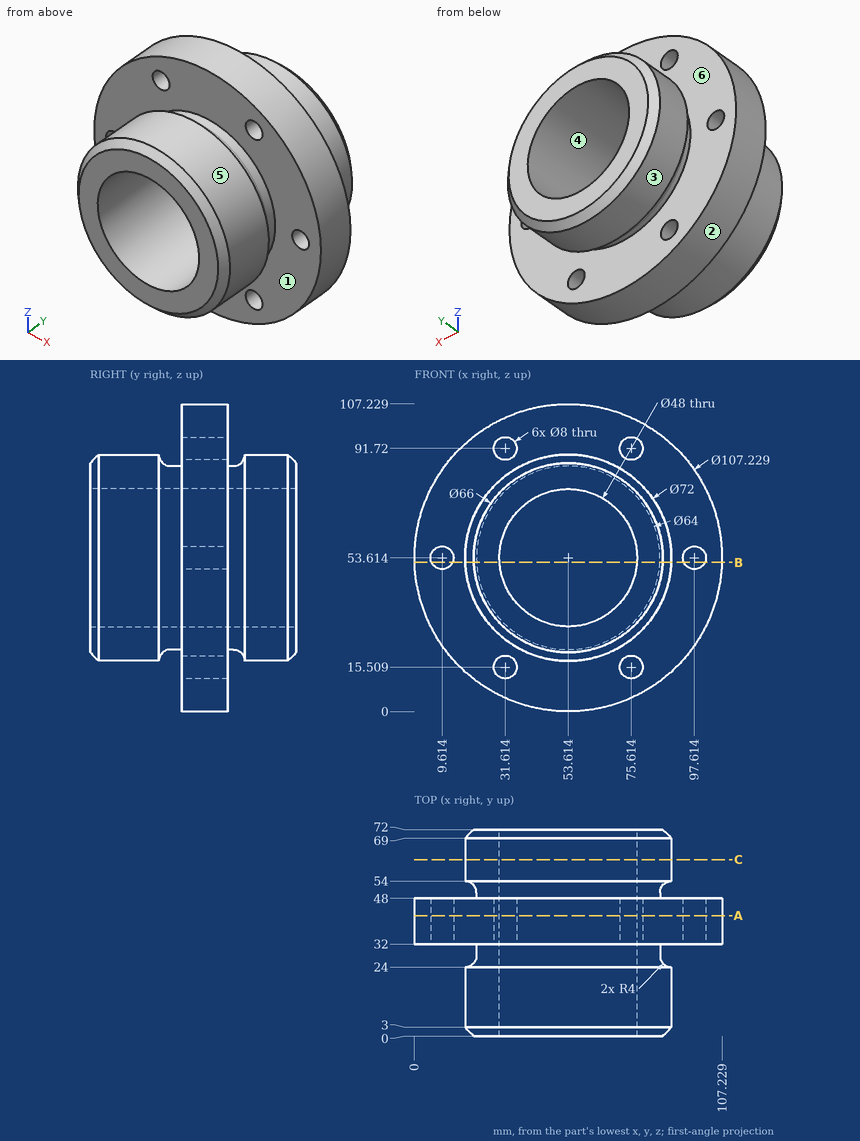
Answer from the drawing. Dimensions are ordinates in mm from the lowest x, y and z of the part. A direction names the side the tool comes from. Coordinates: 2 decimals unless noted, no trailing zeros. Loops run counter-clockwise (first coordinate to the right, second up) from the corner with the lowest first, then second, coordinate; pieces in that order, holes last. Notation, with made-up numbers: (69, 56.25) -> (85, 56.25) arc R21 cw to (85, 70.25) -> close; hole circle Ø3 at (83, 54). An arc over 180 degrees is marked (long way). Return JSON: item names as keys, results as strings.
Item 1: Find the intervals of material crossed by probe 1 along Z at (x, y) = (33, 33) (1 decimal); probe 2 along Y at (x, z) = (9.5, 60.5); probe 3 along X at (y, z) = (7.5, 46.5) (1 decimal), in increasing order.
Answers:
{"probe 1": "z = 4.1 to 11.8, 19.3 to 41.3, 65.9 to 88, 95.5 to 103.1", "probe 2": "y = 32 to 48", "probe 3": "x = 18.3 to 30.7, 76.5 to 88.9"}
Item 2: For the marked faces 1, 2 and 3, determine the directions among +Z, -Z, +X, -X, +Y, -Y from which every point of the face is accessible in a straight line to the end or side of a thin tool.
Answers:
{"face 1": "none", "face 2": "+Y, -Y", "face 3": "+Y"}
Item 3: Find section B-B (z = 52). Count the separate pieces of the cut face and the enclosed holes in it, plus the area to 3 significant figures.
Answers:
{"separate pieces": "4", "enclosed holes": "0", "area": "1,940 mm2"}
Item 4: For a pull along Z with two mould halves and no side action, classify the marked faces 4, 5 and 6 as +Z half, -Z half, draft (parallel to the pull), parting line (faces both ways), or undercut.
Answers:
{"face 4": "undercut", "face 5": "parting line", "face 6": "draft"}
Item 5: Find section A-A (y = 42). Determine the outline of the cut face in (x, z) (1 decimal), plus the area to 3 significant figures.
Answers:
{"outline": "circle Ø107.2 at (53.6, 53.6); hole circle Ø8 at (9.6, 53.6); hole circle Ø8 at (31.6, 15.5); hole circle Ø8 at (31.6, 91.7); hole circle Ø48 at (53.6, 53.6); hole circle Ø8 at (75.6, 15.5); hole circle Ø8 at (75.6, 91.7); hole circle Ø8 at (97.6, 53.6)", "area": "6,920 mm2"}
Item 6: Flat-ended cylindrical pins translate along their axes: P1, Ø10.5, axis at x = 75.61, z = 91.72, coming from the +Y side; P2, Ø5, axis at x = 97.61, z = 53.61, coming from the -Y side; P3, Ø6, axis at x = 89, y = 8, coming from the -Z side (1 decimal); P4, Ø2, axis at x = 14.5, z = 56, coming from the -Y side. Find the tip coordinate at first contact, or state that the pin passes through.
Answers:
{"P1": "stops at y = 48", "P2": "passes through", "P3": "stops at z = 37.9", "P4": "stops at y = 32"}
Item 7: Find section C-C (y = 61.5). Determine the outline of the cut face in (x, z) (1 decimal), plus the area to 3 significant figures.
Answers:
{"outline": "circle Ø72 at (53.6, 53.6); hole circle Ø48 at (53.6, 53.6)", "area": "2,260 mm2"}
